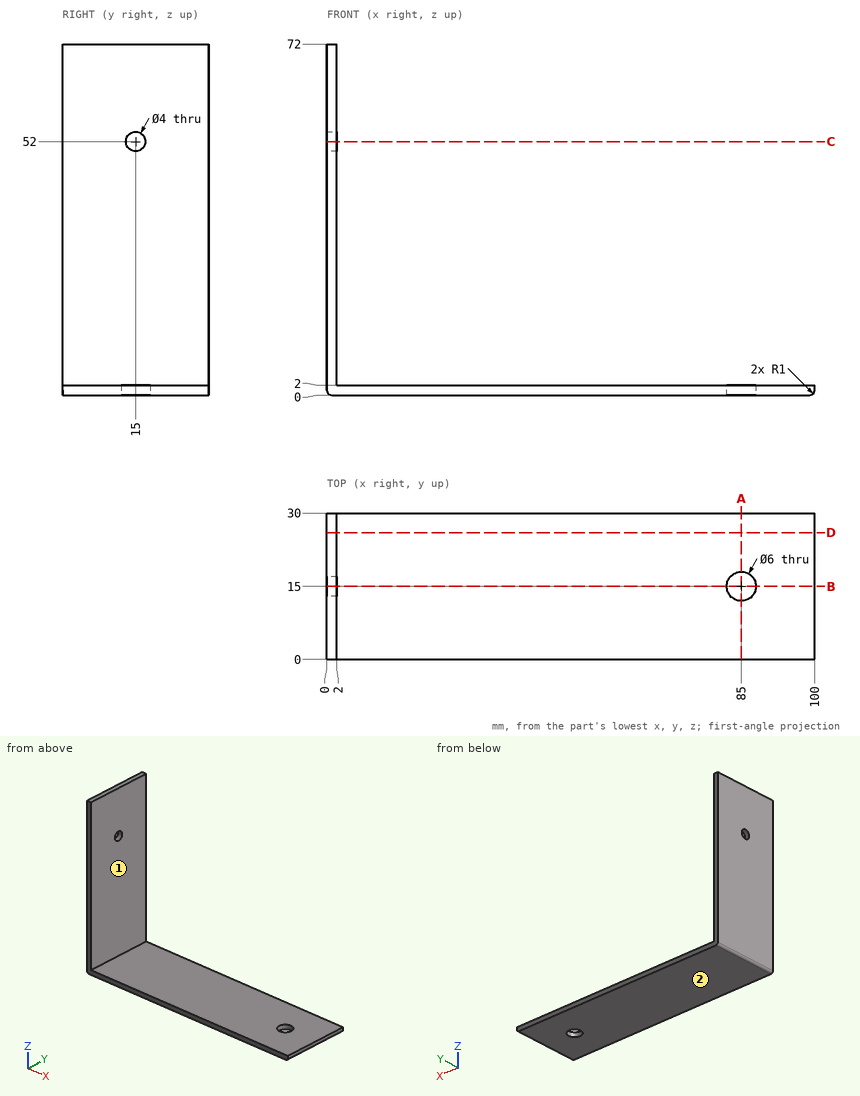
Part print with two shaded views. Sizes in mm from the minimum x, y, z corner. A direction names the side the tool comes from. Round coordinates to 2 decimals unless told otherwise and drop trailing zeros. Loops run counter-clockwise (first coordinate to the right, second up) from the corner with the lowest first, then second, coordinate; pieces in that order, holes last. Notation, with made-up numbers: M 43,-31 L 74,-31 A14 cw 74,-4 Z; hole C 24.5,36 d4. An arc over 180 degrees is marked long. Put each result on its own line as item: value. Start each with the question number.
Item 1: Drill centre lines: line 1 along Y through (x, z) = (0.6, 52); line 2 along Y through (x, z) = (85, 0.8); line 3 along X through (y, z) = (2.75, 37.5). Where is each one in solid material? Low to high.
Item 2: Drop flat-ended pins along their axis: P1, Ø2, axis at x = 44.5, y = 9, coming from the +Z side; P2, Ø2, axis at y = 9.5, z = 31, coming from the +X side. Give the stop position or say it passes through.
Item 3: Cut at D-D (y = 26). List the corners of the cut face in (x, z).
Item 4: Cut at C-C (z = 52). List the corners of the cut face in (x, y), then the cut area to 3 significant figures.
Item 5: Cut at A-A (x = 85). List the corners of the cut face in (y, z).
Item 6: Cut at B-B (y = 15). List the corners of the cut face in (x, z), then the cut area to 3 significant figures.
Item 7: 3-axis set-ups, long thin cutter, end or side, ignore diameter. For the marked faces 1 and 2: which of +Z, -Z, +X, -X, +Y, -Y reach the whole face in a straight line?
Answer block:
1. line 1: 0 to 13, 17 to 30
1. line 2: 0 to 12, 18 to 30
1. line 3: 0 to 2
2. P1: z = 2
2. P2: x = 2
3. outline: M 0,1 A1 ccw 1,0 L 99,0 A1 ccw 100,1 L 100,2 L 2,2 L 2,72 L 0,72 Z
4. outline: M 0,0 L 2,0 L 2,13 L 0,13 Z; M 0,17 L 2,17 L 2,30 L 0,30 Z
4. area: 52.0 mm2
5. outline: M 0,0 L 12,0 L 12,2 L 0,2 Z; M 18,0 L 30,0 L 30,2 L 18,2 Z
6. outline: M 0,1 A1 ccw 1,0 L 82,0 L 82,2 L 2,2 L 2,50 L 0,50 Z; M 0,54 L 2,54 L 2,72 L 0,72 Z; M 88,0 L 99,0 A1 ccw 100,1 L 100,2 L 88,2 Z
6. area: 320 mm2
7. face 1: +Z, +X, +Y, -Y
7. face 2: -Z, +X, -X, +Y, -Y
